Check sheet for the modelled part. Datum: model origin and axes. Units: mm. A direction names the side the tool comes from. Give positions to 0.01 mm unless a question says otherwise; leave off trailing zeros. Loops run counter-clockwise (first coordinate to the right, second up) from the corner with the lowest first, then second, coordinate; pieces in that order, holes last.
Autodesk Inventor part; units mm, degrees
ref_plane "YZ Plane" through (0, 0, 0) normal (1, 0, 0) x (0, 1, 0)
ref_plane "XZ Plane" through (0, 0, 0) normal (0, 1, 0) x (-1, 0, 0)
ref_plane "XY Plane" through (0, 0, 0) normal (0, 0, 1) x (1, 0, 0)
sketch "Sketch1" plane through (0, 0, 0) normal (0, 0, 1) x (1, 0, 0)
  line L0 (0, 0) -> (75, 0)
  line L1 (75, 0) -> (75, 55)
  line L2 (75, 55) -> (0, 55)
  line L3 (0, 55) -> (0, 0)
  dimension "d0" = 55
  dimension "d1" = 75
extrude "Extrusion1" add sketch "Sketch1" along normal blind 10
sketch "Sketch3" plane through (0, 0, 0) normal (0, -1, 0) x (1, 0, 0)
  line L0 (0, 0) -> (0, 10)
  line L1 (0, 0) -> (75, 0)
  line L2 (75, 0) -> (75, 10)
  point P0 (6, 5)
  point P1 (69, 5)
  dimension "d14" = 6
  dimension "d15" = 6
  dimension "d16" = 5
hole "Hole2" at (6, 0, 5) at (69, 0, 5) direction (0, 1, 0) diameter 3.242 depth 11.8 tip angle 118
sketch "Sketch4" plane through (0, 55, 0) normal (0, 1, 0) x (1, 0, 0)
  line L0 (75, 0) -> (75, -10)
  line L1 (75, 0) -> (0, 0)
  line L2 (0, 0) -> (0, -10)
  point P0 (6, -5)
  point P1 (69, -5)
  dimension "d24" = 5
  dimension "d25" = 6
  dimension "d26" = 6
hole "Hole3" at (6, 55, 5) at (69, 55, 5) direction (0, -1, 0) diameter 3.242 depth 11.8 tip angle 118
properties part number "Sides" material "Aluminum-6061"
(1) Material ranges on line 1 (X direction, y = 4.25, z = 5); line 2 (Z direction, x = 6, y = 50), recorded low to high.
(2) Access from +Z, -Z, +X, -X, +Y, -Y to the whole of each face (thin tool, end or side, straight path). Record for faces 1 (the face through (38, 55, 5)), 2 (the face through (6.986, 49.017, 3.714)), 3 (the face through (70.582, 5.983, 5.351)).
(3) Section check A-A on y = 11. Record the boundary of the cut face in (x, z), plus the area to 3 significant figures.
(4) Gauge pin test, flat ends, axial feed: pin 1 Ø2.5 at (x, z) = (69, 5) entering from -Y; pin 2 Ø6 at (y, z) = (31, 5.5) entering from -X; pin 3 Ø2.5 at (x, z) = (69, 5) entering from +Y; pin 4 Ø3 at (x, z) = (6, 5) entering from +Y. Record the tip position at first contact, or that the pin passes through.
(5) Release check for a two-part mould opening along X. For faces 4 (the face through (37, 0, 5)), 5 (the face through (75, 27, 5)), 6 (the face through (5.829, 42.395, 4.777)) record: pulls with the +X half, pulls with the -X half, needs draft (parallel to the pull), parting line crosses it, or undercut.
Computed values:
1. line 1: x = 0 to 4.38, 7.62 to 67.38, 70.62 to 75
1. line 2: z = 0 to 3.38, 6.62 to 10
2. face 1: +Z, -Z, +X, -X, +Y
2. face 2: +Y
2. face 3: -Y
3. outline: (0, 0) - (75, 0) - (75, 10) - (0, 10) - close; hole circle Ø3.24 at (6, 5); hole circle Ø3.24 at (69, 5)
3. area: 733 mm2
4. pin 1: stops at y = 12.02
4. pin 2: stops at x = 0
4. pin 3: stops at y = 42.98
4. pin 4: stops at y = 43.13
5. face 4: needs draft
5. face 5: pulls with the +X half
5. face 6: undercut
